from build123d import *

# Parameters (mm, degrees)
SKETCH1_W           = 50.8
SKETCH1_H           = 50.8
BOSS_EXTRUDE1_DEPTH = 50.8
SKETCH4_R           = 12.7
CUT_EXTRUDE3_DEPTH  = 2.54
SKETCH5_W           = 38.1
SKETCH5_H           = 38.1
CUT_EXTRUDE5_DEPTH  = 3.175
SKETCH6_W           = 25.4
SKETCH6_H           = 25.4
CUT_EXTRUDE6_DEPTH  = 3.175


with BuildPart() as part:
    # Sketch1 → Boss-Extrude1 (new body)
    with BuildSketch(Plane(origin=(0, 0, 0), x_dir=(1, 0, 0), z_dir=(0, 1, 0))):
        Rectangle(SKETCH1_W, SKETCH1_H)
    extrude(amount=BOSS_EXTRUDE1_DEPTH)

    # Sketch4 → Cut-Extrude3 (cut)
    with BuildSketch(Plane(origin=(25.4, 0, 0), x_dir=(0, 0, -1), z_dir=(1, 0, 0))):
        with Locations((0, 31.75)):
            Circle(SKETCH4_R)
    extrude(amount=-CUT_EXTRUDE3_DEPTH, mode=Mode.SUBTRACT)

    # Sketch5 → Cut-Extrude5 (cut)
    with BuildSketch(Plane(origin=(0, 50.8, 0), x_dir=(1, 0, 0), z_dir=(0, 1, 0))):
        Rectangle(SKETCH5_W, SKETCH5_H)
    extrude(amount=-CUT_EXTRUDE5_DEPTH, mode=Mode.SUBTRACT)

    # Sketch6 → Cut-Extrude6 (cut)
    with BuildSketch(Plane(origin=(0, 47.625, 0), x_dir=(1, 0, 0), z_dir=(0, 1, 0))):
        Rectangle(SKETCH6_W, SKETCH6_H)
    extrude(amount=-CUT_EXTRUDE6_DEPTH, mode=Mode.SUBTRACT)


solid = part.part
Input: part model. Units: mm. Frame: model coordinates. A direction names the side the tool comes from. Give positions to 0.01 mm unless a question says otherwise; leave off trailing zeros. Order: outer loops, then holes, each group sorted by start corner. A loop starts at its lowest first (then second) coordinate and runs counter-clockwise, first axis right, second up. Notation, with made-up numbers: (70.5, 0.25) - (109.5, 0.25) arc R27 cw to (109.5, 18.25) - close; hole circle Ø3 at (51.25, 11). An arc over 180 degrees is marked (long way). Answer as a JSON object with one key per item and string values. Group by question number.
Q1. Mould query, pull axis Y, two halves, no side actions, for faces 3 (the face through (-12.7, 46, 0)), 4 (the face through (0, 0, 0)), 5 (the face through (22.86, 32, 0)), 6 (the face through (24.15, 19.35, 2.75)). Classes: pulls with the +Y half, pulls with the -Y half, needs draft (parallel to the pull), parting line crosses it, or undercut.
Q2. Cut plane B-B, the plane x = -14. Output: boundary loops of the cut face in (y, z) (3 decimals), then the cut area to 3 significant figures.
Q3. Line query: probe 1 along Y at (x, z) = (24.8, 0); probe 2 along X at (y, z) = (26.5, -11); probe 3 along Y at (x, z) = (9.5, 10.5). Output: solid intervals per line, ascending.
Q4. Cut plane C-C, the plane y = 31.75. Output: boundary loops of the cut face in (x, z), then the cut area to 3 significant figures.
Q5. Set-up query: faces 1 (the face through (25.4, 19, -5)), 2 (the face through (0, 49, 19.05)). Return all of +Z, -Z, +X, -X, +Y, -Y with unobstructed straight access to the full face (end or side cutting, diameter ignored); none if empty.
Q6. Cut plane A-A, the plane z = 0. Output: boundary loops of the cut face in (x, y) (3 decimals).
Q7. First-contact query: pin 1 Ø20.5 at (x, z) = (-6, 1) entering from +Y (3 decimals); pin 2 Ø3 at (x, z) = (12.5, -1) entering from -Y. Flat tips, straight axial feed; report the tip coordinate or a pass-through.
Q8. Cut plane D-D, the plane z = 9. Output: boundary loops of the cut face in (x, y) (3 decimals).
Results:
{
 "1": {"face 3": "needs draft", "face 4": "pulls with the -Y half", "face 5": "undercut", "face 6": "undercut"},
 "2": {"outline": "(0, -25.4) - (50.8, -25.4) - (50.8, -19.05) - (47.625, -19.05) - (47.625, 19.05) - (50.8, 19.05) - (50.8, 25.4) - (0, 25.4) - close", "area": "2,460 mm^2"},
 "3": {"probe 1": "0 to 19.05, 44.45 to 50.8", "probe 2": "-25.4 to 22.86", "probe 3": "0 to 44.45"},
 "4": {"outline": "(-25.4, -25.4) - (25.4, -25.4) - (25.4, -12.7) - (22.86, -12.7) - (22.86, 12.7) - (25.4, 12.7) - (25.4, 25.4) - (-25.4, 25.4) - close", "area": "2,520 mm^2"},
 "5": {"face 1": "+Z, -Z, +X, +Y, -Y", "face 2": "+Y"},
 "6": {"outline": "(-25.4, 0) - (25.4, 0) - (25.4, 19.05) - (22.86, 19.05) - (22.86, 44.45) - (25.4, 44.45) - (25.4, 50.8) - (19.05, 50.8) - (19.05, 47.625) - (12.7, 47.625) - (12.7, 44.45) - (-12.7, 44.45) - (-12.7, 47.625) - (-19.05, 47.625) - (-19.05, 50.8) - (-25.4, 50.8) - close"},
 "7": {"pin 1": "y = 47.625", "pin 2": "y = 0"},
 "8": {"outline": "(-25.4, 0) - (25.4, 0) - (25.4, 22.79) - (22.86, 22.79) - (22.86, 40.71) - (25.4, 40.71) - (25.4, 50.8) - (19.05, 50.8) - (19.05, 47.625) - (12.7, 47.625) - (12.7, 44.45) - (-12.7, 44.45) - (-12.7, 47.625) - (-19.05, 47.625) - (-19.05, 50.8) - (-25.4, 50.8) - close"}
}
